Geometry: see drawing. Coordinates: mm, zero at the bounding-box minimum. Coordinates: 2 decimals unless noted, no trailing zeros. Order: outer loops, then holes, each group sorted by start corner. A loop starts at its lowest first (then second) coordinate and runs counter-clockwise, first axis right, second up.
Item 1: Contact query for a flat-ended pin moving along its axis: P1, Ø3, axis at x = 9.52, y = 17.46, coming from the +Z side. Output: stop coordinate, or through.
Item 2: Section B-B on z = 0.5. Return the cut outline in (x, y) (1 decimal), then the cut area to 3 significant figures.
Item 3: Ray query, line 1 (X direction, y = 17, z = 0.5) (1 decimal); line 2 (X direction, y = 18, z = 1.4) (1 decimal); line 3 (Y direction, x = 50.8, z = 0.4) (1 decimal). Return the intervals inside material, ascending.
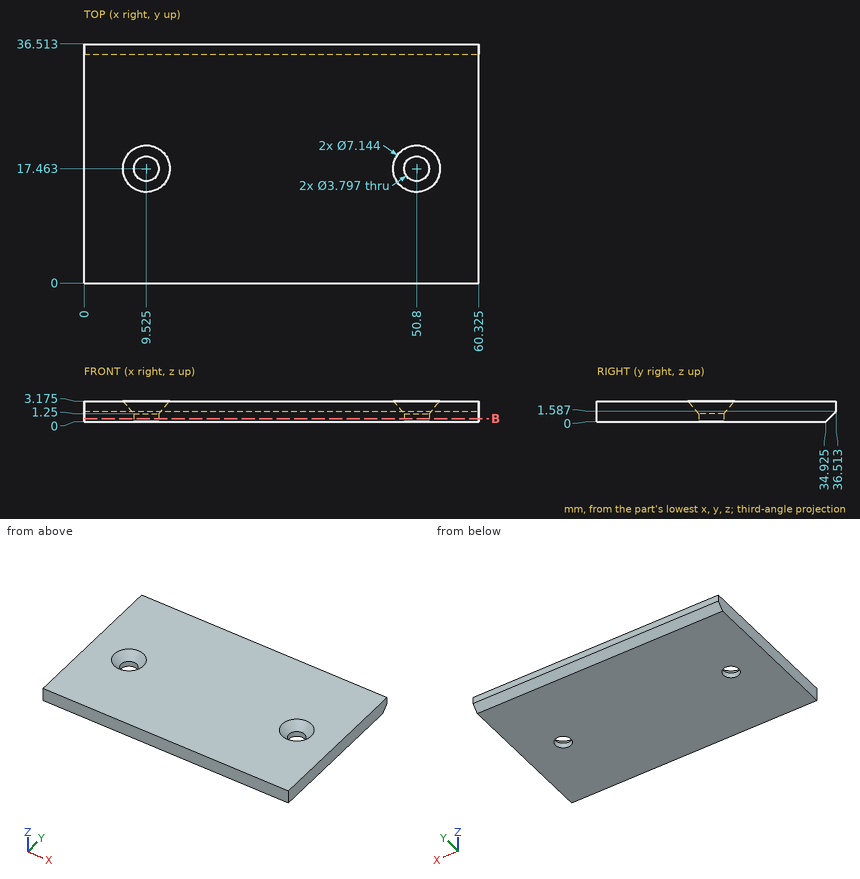
Answer list:
1. P1: passes through
2. outline: (0, 0) - (60.3, 0) - (60.3, 35.4) - (0, 35.4) - close; hole circle Ø3.8 at (9.5, 17.5); hole circle Ø3.8 at (50.8, 17.5)
2. area: 2,110 mm2
3. line 1: x = 0 to 7.7, 11.4 to 49, 52.6 to 60.3
3. line 2: x = 0 to 7.6, 11.5 to 48.8, 52.8 to 60.3
3. line 3: y = 0 to 15.6, 19.4 to 35.3
